Here's how the part is built. I have some questions about the finished solid (model axes, mm). A direction names the side the tool comes from. Coordinates: 2 decimals unless noted, no trailing zeros. Write each loop counter-clockwise with the first axis right and the second up, starting at its lowest first coordinate (ties: lowest second). Pieces come first, ordered by that corner, then holes. Notation, with made-up numbers: M -18.75,41 L 36.25,41 A18 cw 36.25,54 Z; hole C -0.75,17.25 d1. An arc over 180 degrees is marked long. Use a Markdown table: item, result.
```python
from build123d import *

# Parameters (mm, degrees)
MAINBASESKETCH_W          = 15.8
MAINBASESKETCH_H          = 3.2
MAINBASEEXTRUDE_DEPTH     = 7.9
STUDSSKETCH_R             = 2.4
STUDSEXTRUDE_DEPTH        = 1.6
MAINBASESHELL_T           = -1.2
LCUTBLUE_DEPTH            = 19.555463972
LCUTBLUE_DEPTH_BACK       = 19.555463972
CUTADDEDTOLCUT_DEPTH      = 2
MADESLIMCUTSKETCH_W       = 7.9
MADESLIMCUTSKETCH_H       = 7.9
MADESLIMCUT_DEPTH         = 19.897228453
MADESLIMFILLEXT_REACH     = 20.555
SKETCH33_W                = 5.500952983
SKETCH33_H                = 1.199047018
SLIMHOLEEXT_START         = -0.2
SLIMHOLESKETCH_R          = 1.25
SLIMHOLESKETCH_R_2        = 0.75
SLIMHOLEEXT_DEPTH         = 2
ANGLEDSLIMBASECUT_DEPTH   = 19.555463972
ANGLEDSLIMBASESWEEP_DEPTH = 7.9


# Read off the part's stored shape, not the designer's step: AngledSlimBaseSweep
with BuildPart() as part:
    # MainBaseSketch → MainBaseExtrude (new, symmetric)
    with BuildSketch(Plane.XY):
        with Locations((8.581967213, 1.6)):
            Rectangle(MAINBASESKETCH_W, MAINBASESKETCH_H)
    extrude(amount=MAINBASEEXTRUDE_DEPTH, both=True)

    # StudsSketch → StudsExtrude (add)
    with BuildSketch(Plane(origin=(0, 3.2, 0), x_dir=(1, 0, 0), z_dir=(0, 1, 0))):
        with Locations((4.581967213, 4)):
            Circle(STUDSSKETCH_R)
    extrude(amount=STUDSEXTRUDE_DEPTH)

    # MainBaseShell
    mainbaseshell_openings = [part.faces().sort_by_distance(p)[0] for p in [
        (8.581967213, 0, 0),
    ]]
    offset(amount=MAINBASESHELL_T, openings=mainbaseshell_openings, kind=Kind.INTERSECTION)

    # LCUTBlueSketch → LCutBlue (cut, two sides: drawn at the far end of the back side and taken through both)
    with BuildSketch(Plane(origin=(0, 3.2, 0), x_dir=(1, 0, 0), z_dir=(0, 1, 0)).offset(-LCUTBLUE_DEPTH_BACK)):
        Polygon((8.581967213, 53.229874044), (8.581967213, 7.9), (8.581967213, 0), (16.481967213, 0), (61.811841258, 0), (125.917963912, 64.106122654), (72.688089868, 117.335996699), align=None)
    extrude(amount=LCUTBLUE_DEPTH + LCUTBLUE_DEPTH_BACK, mode=Mode.SUBTRACT)

    # CutAddedtoLSketch → CutAddedToLCut (add)
    with BuildSketch(Plane.XZ):
        Polygon((7.382920196, -6.7), (8.581967213, -6.7), (8.581967213, 0), (15.281967213, 0), (15.281967213, 1.199047018), (7.382920196, 1.199047018), (7.382920196, 0), align=None)
    extrude(amount=-CUTADDEDTOLCUT_DEPTH)

    # MadeSlimCutSketch → MadeSlimCut (cut, through all)
    with BuildSketch(Plane.XZ):
        with Locations((4.631967213, -3.95)):
            Rectangle(MADESLIMCUTSKETCH_W, MADESLIMCUTSKETCH_H)
    extrude(amount=-MADESLIMCUT_DEPTH, mode=Mode.SUBTRACT)

    # Sketch33 → MadeSlimFillExt (add, up to next)
    with BuildSketch(Plane.XZ, mode=Mode.PRIVATE) as madeslimfillext_sk1:
        with Locations((4.632443704, 0.599523509)):
            Rectangle(SKETCH33_W, SKETCH33_H)
    madeslimfillext_tool1 = extrude(madeslimfillext_sk1.sketch, amount=-MADESLIMFILLEXT_REACH, mode=Mode.PRIVATE) - part.part
    add(madeslimfillext_tool1.solids().sort_by_distance((4.632444, 0, 0.599524))[0])

    # SlimHoleSketch → SlimHoleExt (add)
    with BuildSketch(Plane.XZ.offset(-2).offset(SLIMHOLEEXT_START)):
        with Locations((8.581967213, 4)):
            Circle(SLIMHOLESKETCH_R)
        with Locations((8.581967213, 4)):
            Circle(SLIMHOLESKETCH_R_2, mode=Mode.SUBTRACT)
    extrude(amount=SLIMHOLEEXT_DEPTH)

    # AngledSlimBaseSketch → AngledSlimBaseCut (cut, through all)
    with BuildSketch(Plane.XY.offset(7.9)):
        Polygon((0.681967213, 2.247699421), (16.481967213, 2.247699421), (16.481967213, 6.15), (0.681967213, 3.2), align=None)
    extrude(amount=-ANGLEDSLIMBASECUT_DEPTH, mode=Mode.SUBTRACT)

    # AngledSlimBaseSweep outline → AngledSlimBaseSweep (add)
    with BuildSketch(Plane.XY):
        Polygon((16.481967213, 2.247699421), (16.481967213, 6.15), (0.681967213, 3.2), (0.681967213, 2.247699421), align=None)
    extrude(amount=ANGLEDSLIMBASESWEEP_DEPTH)


solid = part.part
```
1. Suppose I cut it at D-D on z = 1.5. Write out the boundary of the cut face in (x, y), and give its area (3 significant figures).
Answers follow:
| item | result |
|---|---|
| outline | M 0.68,0 L 1.88,0 L 1.88,2 L 15.28,2 L 15.28,0 L 16.48,0 L 16.48,6.15 L 0.68,3.2 Z |
| area | 47.1 mm2 |
2. We'd pull the mould along Z, two halves only. Please class faces 3 (the face through (8, 2, 0)), 4 (the face through (8, 2, 7.9)), 5 (the face through (10, 2, 4)): +Z half, -Z half, draft (parallel to the pull), parting line (faces both ways), or undercut.
Answers follow:
| item | result |
|---|---|
| face 3 | -Z half |
| face 4 | +Z half |
| face 5 | undercut |
3. Which directions (+Z, -Z, +X, -X, +Y, -Y) give clear straight access to the entire face, cutting with the end or side of a thin tool? Please do faces 1 (the face through (8, 1, 1.199)), 2 (the face through (8.5, 0, 0.5)).
Answers follow:
| item | result |
|---|---|
| face 1 | -Y |
| face 2 | +Z, -Z, +X, -X, -Y |
4. Suppose I cut it at B-B on z = 4. Write out the boundary of the cut face in (x, y).
Answers follow:
| item | result |
|---|---|
| outline | M 0.68,0 L 1.88,0 L 1.88,2 L 7.33,2 L 7.33,0.2 L 7.83,0.2 L 7.83,2 L 9.33,2 L 9.33,0.2 L 9.83,0.2 L 9.83,2 L 15.28,2 L 15.28,0 L 16.48,0 L 16.48,6.15 L 0.68,3.2 Z |
5. Suppose I cut it at A-A on y = 1. Write out the boundary of the cut face in (x, z), and give its area (3 significant figures).
Answers follow:
| item | result |
|---|---|
| outline | M 0.68,0 L 16.48,0 L 16.48,7.9 L 0.68,7.9 Z; C 8.58,4 d2.5; hole M 1.88,1.2 L 15.28,1.2 L 15.28,6.7 L 1.88,6.7 Z; hole C 8.58,4 d1.5 |
| area | 54.2 mm2 |
6. Will this pin go through, and if not, where does the flat tip stop? pin 1 Ø1.2 at (x, z) = (9, 3.5) entering from -Y.
Answers follow:
| item | result |
|---|---|
| pin 1 | stops at y = 0.2 |
7. I need wall thicknesses on probe 1 along X at (y, z) = (1.35, 4); probe 2 along X at (y, z) = (1.5, 6.25); probe 3 along Z at (x, y) = (8.75, 1). Which ranges of each line are inside material? Lowest first, please.
Answers follow:
| item | result |
|---|---|
| probe 1 | x = 0.68 to 1.88, 7.33 to 7.83, 9.33 to 9.83, 15.28 to 16.48 |
| probe 2 | x = 0.68 to 1.88, 15.28 to 16.48 |
| probe 3 | z = 0 to 1.2, 2.76 to 3.27, 4.73 to 5.24, 6.7 to 7.9 |
8. Suppose I cut it at C-C on x = 13.5. Write out the boundary of the cut face in (y, z).
Answers follow:
| item | result |
|---|---|
| outline | M 0,0 L 5.59,0 L 5.59,7.9 L 0,7.9 L 0,6.7 L 2,6.7 L 2,1.2 L 0,1.2 Z |
